For this review, take the finished solid that the model builds, in its own axes (mm). A direction names the side the tool comes from. Round coordinates to 2 decimals unless told otherwise and drop trailing zeros. Order: outer loops, then holes, each group sorted by start corner. A loop starts at its lowest first (then second) coordinate and runs counter-clockwise, first axis right, second up. Notation, with made-up numbers: (33, 60) -> (80, 60) arc R30 ccw to (80, 83) -> close; hole circle Ø3 at (74, 12.5). An arc over 180 degrees is marked (long way). Answer in a Markdown table with one row per item.
```python
from build123d import *

# Parameters (mm, degrees)
SKETCH1_R           = 28.9052
SKETCH1_R_2         = 2.8067
SKETCH1_R_3         = 18.7452
BOSS_EXTRUDE1_DEPTH = 6.35
SHELL1_T            = -2.54
FILLET1_R           = 2.54


with BuildPart() as part:
    # Sketch1 → Boss-Extrude1 (new body)
    with BuildSketch(Plane.XY):
        Circle(SKETCH1_R)
        with Locations((0, 23.8252)):
            Circle(SKETCH1_R_2, mode=Mode.SUBTRACT)
        with Locations((20.63322845, 11.9126)):
            Circle(SKETCH1_R_2, mode=Mode.SUBTRACT)
        with Locations((20.63322845, -11.9126)):
            Circle(SKETCH1_R_2, mode=Mode.SUBTRACT)
        with Locations((0, -23.8252)):
            Circle(SKETCH1_R_2, mode=Mode.SUBTRACT)
        with Locations((-20.63322845, -11.9126)):
            Circle(SKETCH1_R_2, mode=Mode.SUBTRACT)
        with Locations((-20.63322845, 11.9126)):
            Circle(SKETCH1_R_2, mode=Mode.SUBTRACT)
        Circle(SKETCH1_R_3, mode=Mode.SUBTRACT)
    extrude(amount=BOSS_EXTRUDE1_DEPTH)

    # Shell1
    shell1_openings = [part.faces().sort_by_distance(p)[0] for p in [
        (-28.087637483, 0, 6.35),
    ]]
    offset(amount=SHELL1_T, openings=shell1_openings)

    # Fillet1
    fillet1_edges = [part.edges().sort_by_distance(p)[0] for p in [
        (20.242549419, -6.580192403, 4.445),
        (15.819888492, -14.240465833, 4.445),
        (24.894348466, -8.683040107, 4.445),
        (19.966907548, -17.217618129, 4.445),
        (24.894348466, 8.683040107, 4.445),
        (19.966907548, 17.217618129, 4.445),
        (20.242549419, 6.580192403, 4.445),
        (15.819888492, 14.240465833, 4.445),
        (-4.927440918, -25.900658236, 4.445),
        (4.927440918, -25.900658236, 4.445),
        (-4.422660927, -20.820658236, 4.445),
        (4.422660927, -20.820658236, 4.445),
        (-24.894348466, -8.683040107, 4.445),
        (-19.966907548, -17.217618129, 4.445),
        (-20.242549419, -6.580192403, 4.445),
        (-15.819888492, -14.240465833, 4.445),
        (-24.894348466, 8.683040107, 4.445),
        (-19.966907548, 17.217618129, 4.445),
        (-20.242549419, 6.580192403, 4.445),
        (-15.819888492, 14.240465833, 4.445),
        (-4.422660927, 20.820658236, 4.445),
        (4.422660927, 20.820658236, 4.445),
        (-4.927440918, 25.900658236, 4.445),
        (4.927440918, 25.900658236, 4.445),
    ]]
    fillet(fillet1_edges, radius=FILLET1_R - 0.0001)  # a hair under: the kernel refuses the full size


solid = part.part
```
Q1. Take a section at C-C, the plane x = -11. Write out the cut boundary in (y, z).
Answer key:
| item | result |
|---|---|
| outline | (-26.73, 0) -> (-15.18, 0) -> (-15.18, 6.35) -> (-18.22, 6.35) -> (-18.22, 2.54) -> (-23.96, 2.54) -> (-23.96, 6.35) -> (-26.73, 6.35) -> close; (15.18, 0) -> (26.73, 0) -> (26.73, 6.35) -> (23.96, 6.35) -> (23.96, 2.54) -> (18.22, 2.54) -> (18.22, 6.35) -> (15.18, 6.35) -> close |
Q2. Take a section at A-A, the plane y = 0. Write out the cut boundary in (x, z), then the cut area to 3 significant figures.
Answer key:
| item | result |
|---|---|
| outline | (-28.91, 0) -> (-18.75, 0) -> (-18.75, 6.35) -> (-21.29, 6.35) -> (-21.29, 2.54) -> (-26.37, 2.54) -> (-26.37, 6.35) -> (-28.91, 6.35) -> close; (18.75, 0) -> (28.91, 0) -> (28.91, 6.35) -> (26.37, 6.35) -> (26.37, 2.54) -> (21.29, 2.54) -> (21.29, 6.35) -> (18.75, 6.35) -> close |
| area | 90.3 mm^2 |
Q3. Take a section at D-D, the plane z = 1.25. Write out the cut boundary in (x, y).
Answer key:
| item | result |
|---|---|
| outline | circle Ø57.81 at (0, 0); hole circle Ø5.61 at (-20.63, -11.91); hole circle Ø5.61 at (-20.63, 11.91); hole circle Ø37.49 at (0, 0); hole circle Ø5.61 at (0, -23.83); hole circle Ø5.61 at (0, 23.83); hole circle Ø5.61 at (20.63, -11.91); hole circle Ø5.61 at (20.63, 11.91) |
Q4. Clearance check with flat-ended pins moving along their axes: pin 1 Ø1.7 at (x, y) = (23.5, 3) entering from +Z; pin 2 Ø1.5 at (y, z) = (-10.5, 5.5) entering from -X; pin 3 Ø1 at (x, z) = (8.5, 4) entering from -Y; pin 4 Ø5 at (x, y) = (20.63, -11.91) entering from +Z. State where each tip first meets the part, or that it passes through.
Answer key:
| item | result |
|---|---|
| pin 1 | stops at z = 2.54 |
| pin 2 | stops at x = -27.21 |
| pin 3 | stops at y = -27.78 |
| pin 4 | passes through |
Q5. To check wall thickness, follow probe 1 along Y at (x, z) = (0, 1.75); probe 2 along Y at (x, z) = (8.5, 4.75); probe 3 along Y at (x, z) = (20, 3). State the ranges of each line that lie inside material, in increasing order.
Answer key:
| item | result |
|---|---|
| probe 1 | y = -28.91 to -26.63, -21.02 to -18.75, 18.75 to 21.02, 26.63 to 28.91 |
| probe 2 | y = -27.63 to -24.96, -19.51 to -16.71, 16.71 to 19.51, 24.96 to 27.63 |
| probe 3 | y = -20.87 to -14.65, -9.18 to 9.18, 14.65 to 20.87 |
Q6. Take a section at B-B, the plane x = 0. Write out the cut boundary in (y, z), then the cut area to 3 significant figures.
Answer key:
| item | result |
|---|---|
| outline | (-28.91, 0) -> (-26.63, 0) -> (-26.63, 6.35) -> (-28.91, 6.35) -> close; (-21.02, 0) -> (-18.75, 0) -> (-18.75, 6.35) -> (-21.02, 6.35) -> close; (18.75, 0) -> (21.02, 0) -> (21.02, 6.35) -> (18.75, 6.35) -> close; (26.63, 0) -> (28.91, 0) -> (28.91, 6.35) -> (26.63, 6.35) -> close |
| area | 57.7 mm^2 |
Q7. Tool access review of faces 4 (the face through (23.226, 10.838, 3.131)), 5 (the face through (-13.12, 22.87, 4.42)): name each direction out of +Z, -Z, +X, -X, +Y, -Y from which nothing blocks a thin tool from reaching the whole face with its end or side.
Answer key:
| item | result |
|---|---|
| face 4 | +Z, -Z |
| face 5 | +Z |
Q8. The part is to be moulded in two halves that separate along Y. For faces 1 (the face through (-28.877, 1.271, 3.131)), 2 (the face through (0, -19, 0)), 3 (the face through (10.7, 18.4, 4.4)), say which applies: +Y half, -Y half, draft (parallel to the pull), parting line (faces both ways), or undercut.
Answer key:
| item | result |
|---|---|
| face 1 | parting line |
| face 2 | draft |
| face 3 | undercut |
